Check sheet for the modelled part. Datum: model origin and axes. Units: mm. Give positions to 0.01 mm unless a question says otherwise; leave off trailing zeros. Order: outer loops, then holes, each group sorted by start corner. A loop starts at its lowest first (then second) coordinate and runs counter-clockwise, first axis right, second up.
from build123d import *

# Parameters (mm, degrees)
BOSS_EXTRUDE1_DEPTH = 1.34
SKETCH2_R           = 0.25
CUT_EXTRUDE1_DEPTH  = 9.309368207


with BuildPart() as part:
    # Sketch1 → Boss-Extrude1 (new body)
    with BuildSketch(Plane(origin=(0, 0, 0), x_dir=(1, 0, 0), z_dir=(0, 1, 0))):
        with BuildLine():
            ThreePointArc((-5.704564394, 5), (-5.825735931, 4.325735931), (-6.5, 4.204564394))
            Line((-6.5, 4.204564394), (-6.5, -4.204564394))
            ThreePointArc((-6.5, -4.204564394), (-5.825735931, -4.325735931), (-5.704564394, -5))
            Line((-5.704564394, -5), (6.5, -5))
            Line((6.5, -5), (6.5, 5))
            Line((6.5, 5), (-5.704564394, 5))
        make_face()
    extrude(amount=BOSS_EXTRUDE1_DEPTH)

    # Sketch2 → Cut-Extrude1 (cut, through all)
    with BuildSketch(Plane(origin=(0, 1.34, 0), x_dir=(1, 0, 0), z_dir=(0, 1, 0))):
        with Locations(Location((-5, 1.9, 0), (0, 0, 270))):
            Circle(SKETCH2_R)
        with Locations(Location((-5, 0.4, 0), (0, 0, 270))):
            Circle(SKETCH2_R)
        with Locations(Location((-5, -1.1, 0), (0, 0, 270))):
            Circle(SKETCH2_R)
        with Locations(Location((5, 3.5, 0), (0, 0, 270))):
            Circle(SKETCH2_R)
        with Locations(Location((5, -3.5, 0), (0, 0, 270))):
            Circle(SKETCH2_R)
        with Locations(Location((3, -3.5, 0), (0, 0, 270))):
            Circle(SKETCH2_R)
        with Locations(Location((1.5, -3.5, 0), (0, 0, 270))):
            Circle(SKETCH2_R)
        with Locations(Location((-3.4, -3.5, 0), (0, 0, 270))):
            Circle(SKETCH2_R)
    extrude(amount=-CUT_EXTRUDE1_DEPTH, mode=Mode.SUBTRACT)


solid = part.part
1) Material ranges on L1, parallel to X at y = 0.7, z = 3.5; L2, parallel to X at y = 0.6, z = -1.9; L3, parallel to X at y = 0.9, z = -3.5, recorded low to high.
Recorded:
L1: x = -6.5 to -3.65, -3.15 to 1.25, 1.75 to 2.75, 3.25 to 4.75, 5.25 to 6.5
L2: x = -6.5 to -5.25, -4.75 to 6.5
L3: x = -6.5 to 4.75, 5.25 to 6.5
2) Draft check along X on faces 1 (the face through (-6.5, 1, 0)), 2 (the face through (-5.82, 0.66, -4.33)), 3 (the face through (6.5, 1, 0)). Enter one of: +X half, -X half, draft (parallel to the pull), parting line (faces both ways), or undercut.
Recorded:
face 1: -X half
face 2: undercut
face 3: +X half
3) Section check A-A, the plane x = 1.5. Record the cut outline in (y, z).
Recorded:
outline: (0, -5) - (1.34, -5) - (1.34, 3.25) - (0, 3.25) - close; (0, 3.75) - (1.34, 3.75) - (1.34, 5) - (0, 5) - close
4) Section check D-D, the plane x = -5. Record the cut outline in (y, z), then the cut area to 3 significant figures.
Recorded:
outline: (0, -5) - (1.34, -5) - (1.34, -2.15) - (0, -2.15) - close; (0, -1.65) - (1.34, -1.65) - (1.34, -0.65) - (0, -0.65) - close; (0, -0.15) - (1.34, -0.15) - (1.34, 0.85) - (0, 0.85) - close; (0, 1.35) - (1.34, 1.35) - (1.34, 5) - (0, 5) - close
area: 11.4 mm2
5) Section check C-C, the plane z = -3.5. Record the cut outline in (x, y).
Recorded:
outline: (-6.5, 0) - (4.75, 0) - (4.75, 1.34) - (-6.5, 1.34) - close; (5.25, 0) - (6.5, 0) - (6.5, 1.34) - (5.25, 1.34) - close
6) Section check B-B, the plane y = 0.6. State how many separate pieces and enclosed holes the cut face has, then the cut area to 3 significant figures.
Recorded:
separate pieces: 1
enclosed holes: 8
area: 127 mm2
